Part model, mm, in its own coordinate system. A direction names the side the tool comes from. Round coordinates to 2 decimals unless told otherwise and drop trailing zeros. Order: outer loops, then holes, each group sorted by start corner. A loop starts at its lowest first (then second) coordinate and runs counter-clockwise, first axis right, second up. Notation, with made-up numbers: (38, -27.5) - (58, -27.5) arc R28 ccw to (58, 10.5) - close; hole circle Ø5 at (76.5, 27). An arc over 180 degrees is marked (long way). Answer as a JSON object with one key per item and string values.
Solid Edge part; units mm, degrees
sketch "Sketch1" plane through (0, 0, 0) normal (0, 0, 1) x (1, 0, 0)
  circle A0 centre (0, 0) radius 19.5
extrude "Protrusion1" add sketch "Sketch1" along normal blind 16
sketch "Sketch2" plane through (0, 0, 0) normal (0, 0, -1) x (0, -1, 0)
  circle A0 centre (0, 0) radius 14.5
extrude "Cutout1" cut sketch "Sketch2" against normal blind 10
hole "Bohrung_1" at (0, 0, 16) direction (0, 0, -1) diameter 5.3 end up to next
Item 1: Drop flat-ended pins along their axis: P1, Ø5, axis at x = 0, y = 13, coming from the -Z side; P2, Ø2, axis at y = -2, z = 14, coming from the +X side; P3, Ø1.5, axis at x = 8, z = 14.5, coming from the -Y side; P4, Ø2, axis at x = 7.5, y = -1.5, coming from the -Z side. Give the stop position or say it passes through.
Taken from the geometry:
{"P1": "z = 0", "P2": "x = 19.47", "P3": "y = -18.1", "P4": "z = 10"}
Item 2: Cut at A-A (x = 0). Write the cut outline in (y, z), plus the area to 3 significant figures.
Taken from the geometry:
{"outline": "(-19.5, 0) - (-14.5, 0) - (-14.5, 10) - (-2.65, 10) - (-2.65, 16) - (-19.5, 16) - close; (2.65, 10) - (14.5, 10) - (14.5, 0) - (19.5, 0) - (19.5, 16) - (2.65, 16) - close", "area": "302 mm2"}
Item 3: Probe L1, parallel to Y at x = 0, z = 2.75; L2, parallel to Y at x = 0, z = 13.75; L3, parallel to X at y = -0.5, z = 5.25. List the from-to ranges inside material, lowest first. Write a range as from..to.
Taken from the geometry:
{"L1": "-19.5..-14.5, 14.5..19.5", "L2": "-19.5..-2.65, 2.65..19.5", "L3": "-19.49..-14.49, 14.49..19.49"}
Item 4: Tool access for faces 1 (the flat face through (0, -4, 16)), 2 (the flat face through (-3, 0, 10)): list every direction of +Z, -Z, +X, -X, +Y, -Y with a clear straight run to the whole face (end or side of a thin tool).
Taken from the geometry:
{"face 1": "+Z, +X, -X, +Y, -Y", "face 2": "-Z"}
Item 5: Two-plate mould, pull along X, no slides. Class faces 3 (the cylindrical face through (12.864, -6.691, 4.93)), 4 (the cylindrical face through (-2.539, -19.334, 7.888)), 5 (the flat face through (0, 15, 0)): pulls with the +X half, pulls with the -X half, needs draft (parallel to the pull), parting line crosses it, or undercut.
Taken from the geometry:
{"face 3": "undercut", "face 4": "parting line crosses it", "face 5": "needs draft"}
Item 6: Cut at C-C (z = 15). Write the cut outline in (x, y).
Taken from the geometry:
{"outline": "circle Ø39 at (0, 0); hole circle Ø5.3 at (0, 0)"}
Item 7: Cut at D-D (y = -6.5). Write the cut outline in (x, z), plus the area to 3 significant figures.
Taken from the geometry:
{"outline": "(-18.38, 0) - (-12.96, 0) - (-12.96, 10) - (12.96, 10) - (12.96, 0) - (18.38, 0) - (18.38, 16) - (-18.38, 16) - close", "area": "329 mm2"}
